The drawing under review shows one solid part. Ordinate dimensions are in mm from its lowest x, y, z. A direction names the side the tool comes from. Round coordinates to 2 decimals unless told otherwise and drop trailing zeros. Write each loop counter-clockwise with the first axis right and the second up, starting at its lowest first coordinate (ties: lowest second). Pieces come first, ordered by that corner, then holes. Notation, with made-up numbers: M -2,-32 L 17,-32 A11 ccw 17,-19 Z; hole C 43.5,-25 d11. An arc over 180 degrees is marked long. One line per item, written item: value. Start each with the question number.
1) Take a section at A-A, the plane x = 8. Write out the cut boundary in (y, z).
2) Take a section at D-D, the plane z = 1.1. Write out the cut boundary in (x, y), and give its area (3 significant figures).
3) Tool access review of the marked faces 1, 2 and 3: name each direction out of +Z, -Z, +X, -X, +Y, -Y from which nothing blocks a thin tool from reaching the whole face with its end or side.
4) Wall thickness on probe 1 along Z at (x, y) = (1.25, 17.5); probe 2 along X at (y, z) = (15.75, 0.4); probe 3 along Y at (x, z) = (9, 3.25): over which ranges is each line inside the solid? List them lowest first.
5) Take a section at C-C, the plane y = 1.5. Write out the cut boundary in (x, z), and give its area (3 significant figures).
6) Take a section at B-B, the plane z = 2.45. Write out the cut boundary in (x, y), and give its area (3 significant figures).
7) For P1, Ø0.9, axis at x = 1, y = 13, coming from the -Z side; P2, Ø1.5, axis at y = 5, z = 3.5, coming from the -X side; P3, Ø0.6, axis at y = 10, z = 1.5, coming from the +X side; P4, Ø1.6, axis at y = 7.5, z = 0.5, coming from the -X side, all flat-tipped, find the tip position at first contact; note any pin that passes through.
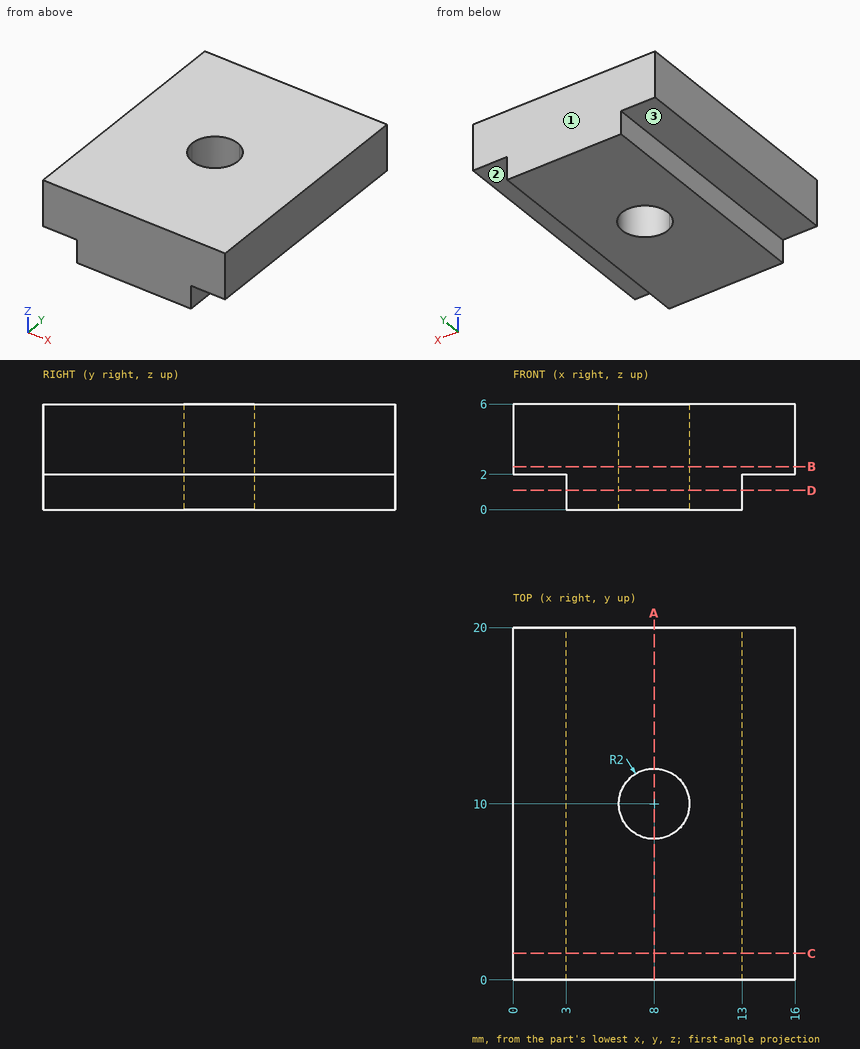
Checked values:
1. outline: M 0,0 L 8,0 L 8,6 L 0,6 Z; M 12,0 L 20,0 L 20,6 L 12,6 Z
2. outline: M 3,0 L 13,0 L 13,20 L 3,20 Z; hole C 8,10 d4
2. area: 187 mm2
3. face 1: +Z, -Z, +X, -X, +Y
3. face 2: -Z, +X, +Y, -Y
3. face 3: -Z, -X, +Y, -Y
4. probe 1: z = 2 to 6
4. probe 2: x = 3 to 13
4. probe 3: y = 0 to 8.27, 11.73 to 20
5. outline: M 0,2 L 3,2 L 3,0 L 13,0 L 13,2 L 16,2 L 16,6 L 0,6 Z
5. area: 84.0 mm2
6. outline: M 0,0 L 16,0 L 16,20 L 0,20 Z; hole C 8,10 d4
6. area: 307 mm2
7. P1: stops at z = 2
7. P2: stops at x = 0
7. P3: stops at x = 13
7. P4: stops at x = 3
